from build123d import *

# Parameters (mm, degrees)
PAD033_DEPTH          = 11
POLARPATTERN002_COUNT = 19
PAD034_DEPTH          = 13


with BuildPart() as part:
    # Sketch066 → Revolution003 (revolve)
    with BuildSketch(Plane.YZ):
        Polygon((2.5, 0), (7.03, 0), (7.03, 1), (6.03, 1), (6.03, 12), (7.03, 12), (7.03, 13), (2.5, 13), align=None)
    revolve(axis=Axis((0, 0, 0), (0, 0, 1)))

    # Sketch065 → Pad033 (new body)
    with BuildSketch(Plane.XY.offset(1)):
        with BuildLine():
            ThreePointArc((5.78, -0.433013), (6.53, 0), (5.78, 0.433013))
            Line((5.78, 0.433013), (5.78, -0.433013))
        make_face()
    pad033 = extrude(amount=PAD033_DEPTH)

    # PolarPattern002: Pad033 ×19 about axis
    polarpattern002_axis = Axis((0, 0, 1), (0, 0, 1))
    for i in range(1, POLARPATTERN002_COUNT):
        add(pad033.rotate(polarpattern002_axis, i * 360 / POLARPATTERN002_COUNT))

    # Sketch067 → Pad034 (join)
    with BuildSketch(Plane.XY):
        with BuildLine():
            ThreePointArc((2, -1.5), (2.5, 0), (2, 1.5))
            Line((2, 1.5), (2, -1.5))
        make_face()
    extrude(amount=PAD034_DEPTH)


solid = part.part
Can you work these out from the model? Positions are in its coordinate system, mm. A direction names the side the tool comes from. Give positions to 0.01 mm unless a question says otherwise; leave off trailing zeros. Order: outer loops, then holes, each group sorted by start corner. A loop starts at its lowest first (then second) coordinate and runs counter-clockwise, first axis right, second up. Notation, with made-up numbers: M 81,33.5 L 124,33.5 A20 cw 124,61.5 Z; hole C 19.25,-21.75 d3. An arc over 180 degrees is marked long. One line per item, written item: value.
Item 1: Please list where these lines run through material, in increasing order: line 1 (Z direction, x = 4, y = -5.75); line 2 (X direction, y = 0, z = 7.5); line 3 (Y direction, x = -2.25, z = 5).
Verdict:
line 1: 0 to 1, 12 to 13
line 2: -6.03 to -2.5, 2 to 6.53
line 3: -5.99 to -1.09, 1.09 to 5.99
Item 2: If we section it at D-D on y = -2.75: Write out the boundary of the cut face in (x, z).
Verdict:
outline: M -6.47,0 L 6.47,0 L 6.47,1 L 5.37,1 L 5.37,12 L 6.47,12 L 6.47,13 L -6.47,13 L -6.47,12 L -5.79,12 L -5.79,1 L -6.47,1 Z
Item 3: If we section it at A-A on y = 0: Write out the boundary of the cut face in (x, z), and give its area (3 significant figures).
Verdict:
outline: M -7.03,0 L -2.5,0 L -2.5,13 L -7.03,13 L -7.03,12 L -6.03,12 L -6.03,1 L -7.03,1 Z; M 2,0 L 7.03,0 L 7.03,1 L 6.53,1 L 6.53,12 L 7.03,12 L 7.03,13 L 2,13 Z
area: 108 mm2
Item 4: If we section it at B-B on x = 1.5: Write out the boundary of the cut face in (y, z).
Verdict:
outline: M -6.87,0 L -2,0 L -2,13 L -6.87,13 L -6.87,12 L -6.35,12 L -6.35,1 L -6.87,1 Z; M 2,0 L 6.87,0 L 6.87,1 L 6.35,1 L 6.35,12 L 6.87,12 L 6.87,13 L 2,13 Z
Item 5: If we mould it in two halves opening along Y, with no side actions, what happens to faces 4 (the face through (-2.5, 0.1, 6.4)), 5 (the face through (0, -3, 0)), 6 (the face through (-4.414, 4.812, 6.423)), 7 (the face through (0.5, 6.01, 6.58))? For each: pulls with the +Y half, pulls with the -Y half, needs draft (parallel to the pull), parting line crosses it, or undercut.
Verdict:
face 4: undercut
face 5: needs draft
face 6: undercut
face 7: pulls with the +Y half
Item 6: For faces 1 (the face through (-6.03, 0.01, 6.58)), 2 (the face through (-6, -2, 12)), 3 (the face through (0.49, -6.01, 6.58)), which set-ups out of +Z, -Z, +X, -X, +Y, -Y let a thin tool reach every point of the face, with its end or its side?
Verdict:
face 1: -X
face 2: none
face 3: -Y
Item 7: For pin 1 (3 mm diameter, centred on y = -5.5, z = 6, fed in from +X); pin 2 (3 mm diameter, centred on y = -4, z = 5.5, fed in from +X); pin 3 (0.9 mm diameter, centred on y = 0.5, z = 3.5, fed in from -X), each with a flat end and sliding along its axis, tell me the tip position at first contact or that it passes through.
Verdict:
pin 1: x = 5.16
pin 2: x = 5.49
pin 3: x = -6.45
Item 8: If we section it at C-C on x = -4: Write out the boundary of the cut face in (y, z).
Verdict:
outline: M -5.78,0 L 5.78,0 L 5.78,1 L 4.93,1 L 4.93,12 L 5.78,12 L 5.78,13 L -5.78,13 L -5.78,12 L -4.93,12 L -4.93,1 L -5.78,1 Z
